```python
from build123d import *

# Parameters (mm, degrees)
SKETCH1_R           = 50.8
SKETCH1_R_2         = 2.666666667
BOSS_EXTRUDE1_DEPTH = 6.35
CUT_EXTRUDE1_START  = -12.7
CUT_EXTRUDE1_DEPTH  = 12.7
CUT_EXTRUDE2_START  = -17.348
CUT_EXTRUDE2_DEPTH  = 17.348


with BuildPart() as part:
    # Sketch1 → Boss-Extrude1 (new body)
    with BuildSketch(Plane(origin=(0, 0, 0), x_dir=(1, 0, 0), z_dir=(0, 1, 0))):
        with Locations(Location((0, 0, 0), (0, 0, 270))):
            Circle(SKETCH1_R)
        with Locations(Location((0, 0, 0), (0, 0, 270))):
            Circle(SKETCH1_R_2, mode=Mode.SUBTRACT)
    extrude(amount=BOSS_EXTRUDE1_DEPTH)

    # Sketch2 → Cut-Extrude1 (cut)
    with BuildSketch(Plane(origin=(0, 6.35, 0), x_dir=(1, 0, 0), z_dir=(0, 1, 0)).offset(CUT_EXTRUDE1_START)):
        with BuildLine():
            ThreePointArc((50.8, 0), (47.519048812, 17.960512242), (38.1, 33.601041651))
            Line((38.1, 33.601041651), (38.1, 0))
            Line((38.1, 0), (38.1, -33.601041651))
            ThreePointArc((38.1, -33.601041651), (47.519048812, -17.960512242), (50.8, 0))
        make_face()
        with BuildLine():
            ThreePointArc((-38.1, 33.601041651), (-47.519048812, 17.960512242), (-50.8, 0))
            Line((-50.8, 0), (-38.1, 0))
            Line((-38.1, 0), (-38.1, 33.601041651))
        make_face()
        with BuildLine():
            Line((-38.1, 0), (-50.8, 0))
            ThreePointArc((-50.8, 0), (-47.519048812, -17.960512242), (-38.1, -33.601041651))
            Line((-38.1, -33.601041651), (-38.1, 0))
        make_face()
    extrude(amount=CUT_EXTRUDE1_DEPTH, mode=Mode.SUBTRACT)

    # Sketch3 → Cut-Extrude2 (cut)
    with BuildSketch(Plane(origin=(0, 6.35, 0), x_dir=(1, 0, 0), z_dir=(0, 1, 0)).offset(CUT_EXTRUDE2_START)):
        with BuildLine():
            Line((22.86, 33.601041651), (38.1, 33.601041651))
            ThreePointArc((38.1, 33.601041651), (29.725219859, 41.19528255), (19.87826087, 46.74927534))
            Line((19.87826087, 46.74927534), (22.86, 33.601041651))
        make_face()
        Polygon((38.1, 33.601041651), (22.86, 33.601041651), (38.1, -33.601041651), align=None)
    extrude(amount=CUT_EXTRUDE2_DEPTH, mode=Mode.SUBTRACT)


solid = part.part
```
Source: CAD feature listing. Evaluate the final solid. Frame: model axes, mm. Give positions to 0.01 mm unless a question says otherwise; leave off trailing zeros. Loops run counter-clockwise (first coordinate to the right, second up) from the corner with the lowest first, then second, coordinate; pieces in that order, holes last. Notation, with made-up numbers: (-11, 82.25) -> (19, 82.25) arc R22 ccw to (19, 94.25) -> close; hole circle Ø7 at (9.5, 43). An arc over 180 degrees is marked (long way). Use a Markdown table: item, result. Add a question column.
(1) Section query B-B (x = 0). Output: boundary loops of the cut face in (y, z), then the cut area to 3 significant figures.
(2) Section query A-A (z = 0). Output: boundary loops of the cut face in (x, y), then the cut area to 3 significant figures.
(3) First-contact query: pin 1 Ø2 at (x, y) = (4.5, 4.5) entering from -Z; pin 2 Ø5 at (x, z) = (0, 0) entering from -Y. Flat tips, straight axial feed; report the tip coordinate or a pass-through.
(4) Ray query, line 1 (X direction, y = 4.75, z = 0); line 2 (Z direction, x = 14, y = 0.5); line 3 (X direction, y = 3, z = -37.5). Return the intervals inside material, ascending.
(5) Section query D-D (z = 15.5). Output: boundary loops of the cut face in (x, y), then the cut area to 3 significant figures.
(6) Pull-direction query (X, two-part tool) for faces 1 (the face through (-0.603, 3.131, 50.796)), 2 (the face through (-8, 0, -1)), 3 (the face through (-38.1, 3, 0)), 4 (the face through (0.801, 3.131, 2.544)); classes: +X half, -X half, draft (parallel to the pull), parting line (faces both ways), or undercut.
(7) Section query C-C (y = 3.5). Output: boundary loops of the cut face in (x, z).
Checked values:
| question | item | result |
|---|---|---|
| 1 | outline | (0, -50.8) -> (6.35, -50.8) -> (6.35, -2.67) -> (0, -2.67) -> close; (0, 2.67) -> (6.35, 2.67) -> (6.35, 50.8) -> (0, 50.8) -> close |
| 1 | area | 611 mm^2 |
| 2 | outline | (-38.1, 0) -> (-2.67, 0) -> (-2.67, 6.35) -> (-38.1, 6.35) -> close; (2.67, 0) -> (30.48, 0) -> (30.48, 6.35) -> (2.67, 6.35) -> close |
| 2 | area | 402 mm^2 |
| 3 | pin 1 | z = -50.68 |
| 3 | pin 2 | through |
| 4 | line 1 | -38.1 to -2.67, 2.67 to 30.48 |
| 4 | line 2 | -48.83 to 48.83 |
| 4 | line 3 | -34.27 to 21.98 |
| 5 | outline | (-38.1, 0) -> (34, 0) -> (34, 6.35) -> (-38.1, 6.35) -> close |
| 5 | area | 458 mm^2 |
| 6 | face 1 | parting line |
| 6 | face 2 | draft |
| 6 | face 3 | -X half |
| 6 | face 4 | undercut |
| 7 | outline | (-38.1, -33.6) arc R50.8 ccw to (19.88, -46.75) -> (38.1, 33.6) arc R50.8 ccw to (-38.1, 33.6) -> close; hole circle Ø5.33 at (0, 0) |
